```python
from build123d import *

# Parameters (mm, degrees)
SKETCH_1_W                 = 55
SKETCH_1_H                 = 45
EXTRUDE_360_DEPTH          = 2
CUT_EXTRUDE_614_DEPTH      = 36.587919299
CUT_EXTRUDE_614_DEPTH_BACK = 36.587919299
SKETCH_2_R                 = 1.5
EXTRUDE_883_DEPTH          = 10
EXTRUDE_883_DEPTH_BACK     = 6


with BuildPart() as part:
    # Эскиз1 → Extrude 360 (new body)
    with BuildSketch(Plane(origin=(0, 0, 0), x_dir=(1, 0, 0), z_dir=(0, 1, 0))):
        Rectangle(SKETCH_1_W, SKETCH_1_H)
    extrude(amount=EXTRUDE_360_DEPTH)

    # Эскиз2 → Cut-Extrude 614 (cut, two sides: drawn at the far end of the back side and taken through both)
    with BuildSketch(Plane(origin=(0, 2, 0), x_dir=(1, 0, 0), z_dir=(0, 1, 0)).offset(-CUT_EXTRUDE_614_DEPTH_BACK)):
        with Locations(Location((-25, 20, 0), (0, 0, 270))):
            Circle(SKETCH_2_R)
        with Locations(Location((25, 20, 0), (0, 0, 270))):
            Circle(SKETCH_2_R)
        with Locations(Location((25, -20, 0), (0, 0, 270))):
            Circle(SKETCH_2_R)
        with Locations(Location((-25, -20, 0), (0, 0, 270))):
            Circle(SKETCH_2_R)
    extrude(amount=CUT_EXTRUDE_614_DEPTH + CUT_EXTRUDE_614_DEPTH_BACK, mode=Mode.SUBTRACT)

    # Эскиз3 → Extrude 883 (add, two sides: drawn at the far end of the back side and taken through both)
    with BuildSketch(Plane(origin=(0, 2, 0), x_dir=(1, 0, 0), z_dir=(0, 1, 0)).offset(-EXTRUDE_883_DEPTH_BACK)):
        Polygon((-27.5, 17.5), (-22.5, 17.5), (-22.5, 22.5), (22.5, 22.5), (22.5, 17.5), (27.5, 17.5), (27.5, -17.5), (22.5, -17.5), (22.5, -22.5), (-22.5, -22.5), (-22.5, -17.5), (-27.5, -17.5), align=None)
    extrude(amount=EXTRUDE_883_DEPTH + EXTRUDE_883_DEPTH_BACK)


solid = part.part
```
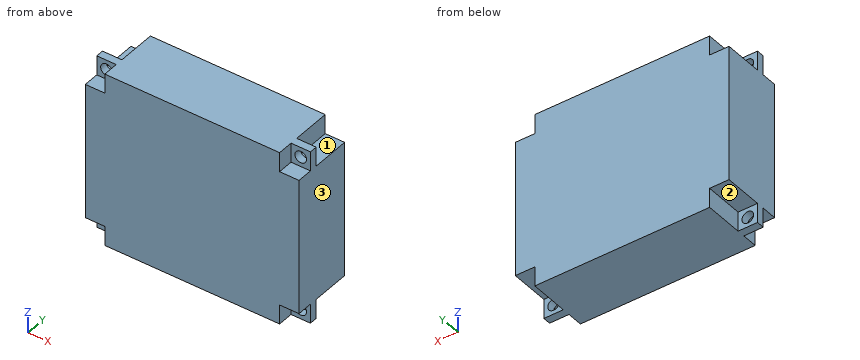
Build history of the part. All positions in model axes, mm. Face numbers are marked on the shaded views. A direction names the side the tool comes from. Round coordinates to 2 decimals unless told otherwise and drop trailing zeros. Write each loop counter-clockwise with the first axis right and the second up, starting at its lowest first coordinate (ties: lowest second). Pieces come first, ordered by that corner, then holes. Notation, with made-up numbers: (33, -4.75) - (65, -4.75) arc R24 ccw to (65, 34.25) - close; hole circle Ø8 at (85, 62). An arc over 180 degrees is marked (long way). Write each question's results on one line, items separated by ' | '. Start each with the question number.
Item 1: Saw through at C-C (y = 5.5). Write the cut outline in (x, z).
Item 2: Drop flat-ended pins along their axis: P1, Ø2.5, axis at y = 5.5, z = -21, coming from the +X side; P2, Ø5.5, axis at x = 25.5, y = 5.5, coming from the -Z side; P3, Ø2, axis at y = -2, z = -20.5, coming from the -X side. Give the stop position or say it passes through.
Item 3: Saw through at A-A (z = -20). Write the cut outline in (x, y).
Item 4: Wall check: L1, parallel to Z at x = 25, y = 0.75; L2, parallel to X at y = 1.45, z = 20. Give the ranges that are in metal, low to high. Write a range as [from, to].
Item 5: Which spindle directions (+Z, -Z, +X, -X, +Y, -Y) get a long thin tool onto all of the face, cutting with end or side? Do the marked faces 1, 2 and 3. Say none if no direction does.
Item 6: Saw through at B-B (x = -25). Write the cut outline in (y, z).
Results are:
1) outline: (-27.5, -17.5) - (-22.5, -17.5) - (-22.5, -22.5) - (22.5, -22.5) - (22.5, -17.5) - (27.5, -17.5) - (27.5, 17.5) - (22.5, 17.5) - (22.5, 22.5) - (-22.5, 22.5) - (-22.5, 17.5) - (-27.5, 17.5) - close
2) P1: stops at x = 22.5 | P2: stops at z = -17.5 | P3: stops at x = -22.5
3) outline: (-27.5, 0) - (-26.5, 0) - (-26.5, 2) - (-27.5, 2) - close; (-23.5, 0) - (-22.5, 0) - (-22.5, -4) - (22.5, -4) - (22.5, 0) - (23.5, 0) - (23.5, 2) - (22.5, 2) - (22.5, 12) - (-22.5, 12) - (-22.5, 2) - (-23.5, 2) - close; (26.5, 0) - (27.5, 0) - (27.5, 2) - (26.5, 2) - close
4) L1: z = [-22.5, -21.5], [-18.5, 18.5], [21.5, 22.5] | L2: x = [-27.5, -26.5], [-23.5, 23.5], [26.5, 27.5]
5) face 1: +Z, +X, +Y | face 2: -Z, -X, +Y | face 3: +Z, -Z, +X, +Y, -Y
6) outline: (-4, -17.5) - (0, -17.5) - (0, -18.5) - (2, -18.5) - (2, -17.5) - (12, -17.5) - (12, 17.5) - (2, 17.5) - (2, 18.5) - (0, 18.5) - (0, 17.5) - (-4, 17.5) - close; (0, -22.5) - (2, -22.5) - (2, -21.5) - (0, -21.5) - close; (0, 21.5) - (2, 21.5) - (2, 22.5) - (0, 22.5) - close
